Source: CAD feature listing. Evaluate the final solid. Frame: model axes, mm. Give positions to 0.01 mm unless a question says otherwise; leave off trailing zeros. Order: outer loops, then holes, each group sorted by start corner. A loop starts at its lowest first (then second) coordinate and runs counter-clockwise, first axis right, second up.
from build123d import *

# Parameters (mm, degrees)
SKETCH1_R           = 3.025
BOSS_EXTRUDE1_DEPTH = 2.5


with BuildPart() as part:
    # Sketch1 → Boss-Extrude1 (new body, symmetric)
    with BuildSketch(Plane.XY):
        with BuildLine():
            Line((-15.24, -30.48), (15.24, -30.48))
            Line((15.24, -30.48), (15.24, 0))
            ThreePointArc((15.24, 0), (0, 15.24), (-15.24, 0))
            Line((-15.24, 0), (-15.24, -30.48))
        make_face()
        Circle(SKETCH1_R, mode=Mode.SUBTRACT)
    extrude(amount=BOSS_EXTRUDE1_DEPTH, both=True)


solid = part.part
1) Section query B-B on z = 0.5. Output: boundary loops of the cut face in (x, y) (3 decimals), and give its area (3 significant figures).
Checks:
outline: (-15.24, -30.48) - (15.24, -30.48) - (15.24, 0) arc R15.24 ccw to (-15.24, 0) - close; hole circle Ø6.05 at (0, 0)
area: 1,270 mm2
2) Section query A-A on x = 0. Output: boundary loops of the cut face in (y, z) (3 decimals), and give its area (3 significant figures).
Checks:
outline: (-30.48, -2.5) - (-3.025, -2.5) - (-3.025, 2.5) - (-30.48, 2.5) - close; (3.025, -2.5) - (15.24, -2.5) - (15.24, 2.5) - (3.025, 2.5) - close
area: 198 mm2
3) Pull-direction query (Y, two-part tool) for faces 1 (the face through (0, -7, 2.5)), 2 (the face through (0.335, 15.236, 0.035)), 3 (the face through (2.794, -1.159, -0.035)); classes: +Y half, -Y half, draft (parallel to the pull), parting line (faces both ways), or undercut.
Checks:
face 1: draft
face 2: +Y half
face 3: undercut
4) First-contact query: pin 1 Ø1 at (x, z) = (3.5, 1.5) entering from +Y; pin 2 Ø5.5 at (x, y) = (0, 0) entering from -Z. Flat tips, straight axial feed; report the tip coordinate or a pass-through.
Checks:
pin 1: stops at y = 14.94
pin 2: passes through
5) Section query C-C on y = 8. Output: boundary loops of the cut face in (x, z).
Checks:
outline: (-12.97, -2.5) - (12.97, -2.5) - (12.97, 2.5) - (-12.97, 2.5) - close
6) Ray query, L1, parallel to Y at x = 0, z = 1.4 (3 decimals); L2, parallel to X at y = -2, z = 0.75; L3, parallel to Y at x = -1.5, z = -1.6. Return the intervals inside material, ascending.
Checks:
L1: y = -30.48 to -3.025, 3.025 to 15.24
L2: x = -15.24 to -2.27, 2.27 to 15.24
L3: y = -30.48 to -2.63, 2.63 to 15.17
